Read the model definition and answer for the solid it produces. Units are mm, in the model's axes. A direction names the side the tool comes from. Give positions to 0.01 mm unless a question says otherwise; leave off trailing zeros. Loops run counter-clockwise (first coordinate to the right, second up) from the corner with the lowest first, then second, coordinate; pieces in that order, holes last. Notation, with made-up numbers: (78, -7.75) - (103, -7.75) arc R21 cw to (103, 24.25) - close; hole circle Ø10 at (-12.5, -31.5). An arc over 180 degrees is marked (long way). Use a Markdown table: item, result. Add a question column.
Item 1: A cutting plane is placed at B-B (y = 0). Determine the outline of the cut face in (x, z).
Item 2: For a pull along Y with two mould halves and no side action, classify faces 1 (the face through (-1.486, 15, 1)), 2 (the face through (-0.682, -15.962, 1.252)), 3 (the face through (0.184, 4.868, 1.288)) as +Y half, -Y half, draft (parallel to the pull), parting line (faces both ways), or undercut.
Item 3: Consider probe 1 along Y at (x, z) = (2.5, 0.6); probe 2 along X at (y, z) = (-1, 1.7); probe 3 along X at (y, z) = (11, 2.1). Determine where each line is inside the solid, lowest interval first. Write a range as [from, to].
Item 4: A cutting plane is placed at D-D (x = 6). Determine the outline of the cut face in (y, z).
Item 5: A cutting plane is placed at A-A (z = 0.7). Determine the outline of the cut face in (x, y) (3 decimals), plus the area to 3 significant figures.
Item 6: A cutting plane is placed at C-C (y = 8.5). Determine the outline of the cut face in (x, z).
Item 7: Each of these flat-tipped pins is pushed along its axis until it touches: P1, Ø1.3, axis at x = 3.5, z = 1.5, coming from the +Y side; P2, Ø1, axis at y = 15, z = 1, coming from the +X side; P3, Ø1, axis at x = -11, z = 1, coming from the +Y side. Where does it stop, or does it pass through?
Item 8: Which of the six approach directions +Z, -Z, +X, -X, +Y, -Y give full straight-line access (tool end or side, diameter ignored) to faces 4 (the face through (1.486, 15, 1)), 5 (the face through (1.689, 0, 1)), 6 (the face through (0, 0, 0))?
from build123d import *

# Parameters (mm, degrees)
SKETCH1_R           = 15.9766
SKETCH1_W           = 2.9718
SKETCH1_H           = 2.9718
BOSS_EXTRUDE1_DEPTH = 2.54
CUT_EXTRUDE1_DEPTH  = 2.54


with BuildPart() as part:
    # Sketch1 → Boss-Extrude1 (new body)
    with BuildSketch(Plane.XY):
        Circle(SKETCH1_R)
        with Locations((-3.175, 0)):
            Rectangle(SKETCH1_W, SKETCH1_H, mode=Mode.SUBTRACT)
        with Locations((3.175, 0)):
            Rectangle(SKETCH1_W, SKETCH1_H, mode=Mode.SUBTRACT)
    extrude(amount=BOSS_EXTRUDE1_DEPTH)

    # Sketch2 → Cut-Extrude1 (cut)
    with BuildSketch(Plane.XY.offset(2.54)):
        with BuildLine():
            Line((-1.4859, 13.942701891), (-1.4859, 18.9484))
            Line((-1.4859, 18.9484), (1.4859, 18.9484))
            Line((1.4859, 18.9484), (1.4859, 13.942701891))
            ThreePointArc((1.4859, 13.942701891), (0, 4.8641), (-1.4859, 13.942701891))
        make_face()
    extrude(amount=-CUT_EXTRUDE1_DEPTH, mode=Mode.SUBTRACT)


solid = part.part
Geometry says:
| question | item | result |
|---|---|---|
| 1 | outline | (-15.98, 0) - (-4.66, 0) - (-4.66, 2.54) - (-15.98, 2.54) - close; (-1.69, 0) - (1.69, 0) - (1.69, 2.54) - (-1.69, 2.54) - close; (4.66, 0) - (15.98, 0) - (15.98, 2.54) - (4.66, 2.54) - close |
| 2 | face 1 | draft |
| 2 | face 2 | parting line |
| 2 | face 3 | undercut |
| 3 | probe 1 | [-15.78, -1.49], [1.49, 5.59], [13.46, 15.78] |
| 3 | probe 2 | [-15.95, -4.66], [-1.69, 1.69], [4.66, 15.95] |
| 3 | probe 3 | [-11.59, -4.42], [4.42, 11.59] |
| 4 | outline | (-14.81, 0) - (14.81, 0) - (14.81, 2.54) - (-14.81, 2.54) - close |
| 5 | outline | (-1.486, 13.943) - (-1.486, 15.907) arc R15.977 ccw (long way) to (1.486, 15.907) - (1.486, 13.943) arc R4.661 cw (long way) to start; hole (-4.661, -1.486) - (-1.689, -1.486) - (-1.689, 1.486) - (-4.661, 1.486) - close; hole (1.689, -1.486) - (4.661, -1.486) - (4.661, 1.486) - (1.689, 1.486) - close |
| 5 | area | 710 mm² |
| 6 | outline | (-13.53, 0) - (-4.55, 0) - (-4.55, 2.54) - (-13.53, 2.54) - close; (4.55, 0) - (13.53, 0) - (13.53, 2.54) - (4.55, 2.54) - close |
| 7 | P1 | y = 15.72 |
| 7 | P2 | x = 6.71 |
| 7 | P3 | y = 12.04 |
| 8 | face 4 | +Z, -Z, +Y |
| 8 | face 5 | +Z, -Z |
| 8 | face 6 | -Z, +X, -X, +Y, -Y |
